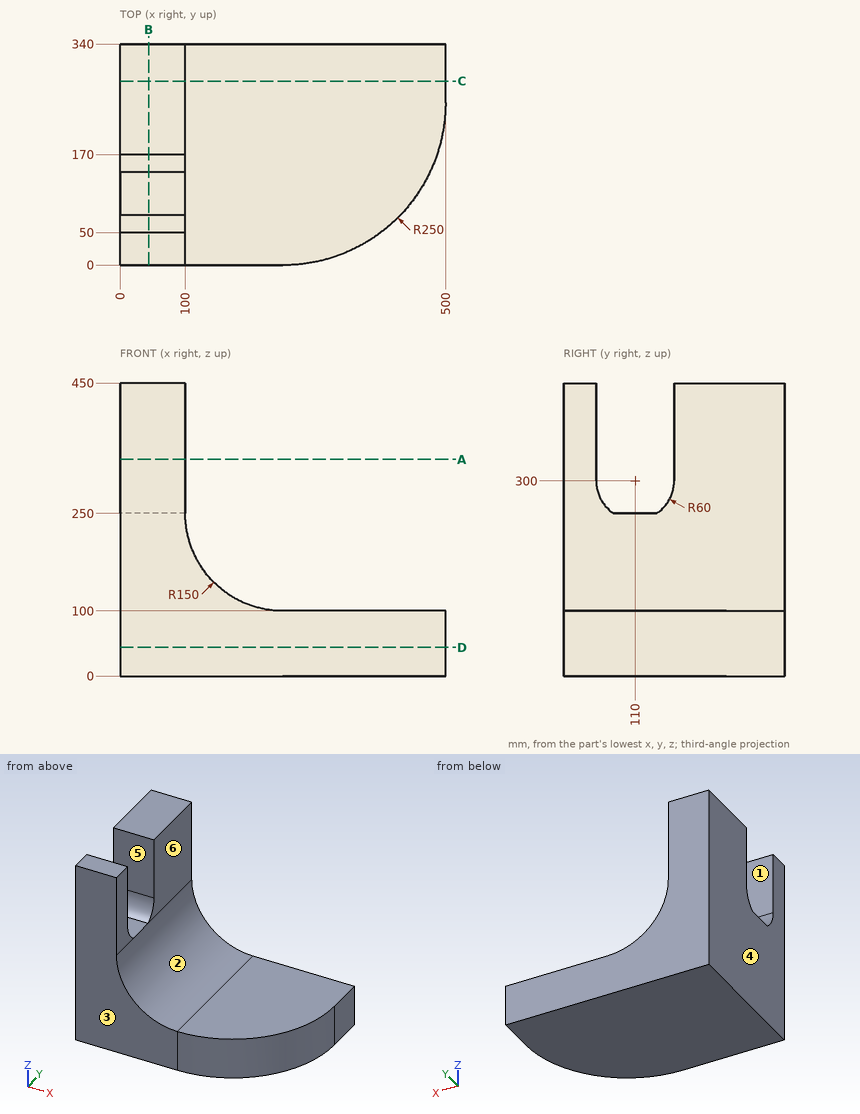
Geometry: see drawing. Coordinates: mm, zero at the bounding-box minimum. A direction names the side the tool comes from. Give positions to 0.01 mm unless a question says otherwise; leave off trailing zeros. Write each loop counter-clockwise with the first axis right and the second up, starting at its lowest first coordinate (ties: lowest second). Pieces come first, ordered by that corner, then holes. Notation, with made-up numbers: M 73.25,75 L 110.25,75 A17 cw 110.25,90 Z; hole C 80.5,71 d9. An arc over 180 degrees is marked long. Return JSON: item names as keys, results as strings. Group by question number.
1) Set-up query: the marked faces 4, 5 and 6. Return all of +Z, -Z, +X, -X, +Y, -Y with unobstructed straight access to the full face (end or side cutting, diameter ignored); none if empty.
2) Ray query, L1, parallel to Y at x = 36.5, z = 364.5; L2, parallel to Z at x = 430.5, y = 164. Return the intervals inside material, ascending.
3) First-contact query: pin 1 Ø4 at (x, y) = (197, 278.5) entering from +Z; pin 2 Ø4 at (y, z) = (36.5, 96) entering from +X; pin 3 Ø12 at (y, z) = (163.5, 342.5) entering from +X. Flat tips, straight axial feed; report the tip coordinate or a pass-through.
4) Draft query along Y for the marked faces 1, 2 and 3. Return one class per face: released by +Y, released by -Y, zero draft, split by the parting line, or undercut.
5) Cut plane B-B, the plane x = 43.5. Output: boundary loops of the cut face in (y, z).
6) Cut plane C-C, the plane y = 283. Output: boundary loops of the cut face in (x, z), then the cut area to 3 significant figures.
7) Cut plane A-A, the plane z = 333. Output: boundary loops of the cut face in (x, y).
8) Cut plane D-D, the plane z = 44. Output: boundary loops of the cut face in (x, y).
Data:
{
 "1": {"face 4": "+Z, -Z, -X, +Y, -Y", "face 5": "+Z, +X, -X", "face 6": "+Z, +X, +Y, -Y"},
 "2": {"L1": "y = 0 to 50, 170 to 340", "L2": "z = 0 to 100"},
 "3": {"pin 1": "stops at z = 110.45", "pin 2": "stops at x = 383.3", "pin 3": "passes through"},
 "4": {"face 1": "undercut", "face 2": "zero draft", "face 3": "released by -Y"},
 "5": {"outline": "M 0,0 L 340,0 L 340,450 L 170,450 L 170,300 A60 cw 143.17,250 L 76.83,250 A60 cw 50,300 L 50,450 L 0,450 Z"},
 "6": {"outline": "M 0,0 L 500,0 L 500,100 L 250,100 A150 cw 100,250 L 100,450 L 0,450 Z", "area": "89,800 mm²"},
 "7": {"outline": "M 0,0 L 100,0 L 100,50 L 0,50 Z; M 0,170 L 100,170 L 100,340 L 0,340 Z"},
 "8": {"outline": "M 0,0 L 250,0 A250 ccw 500,250 L 500,340 L 0,340 Z"}
}
